```python
from build123d import *

# Parameters (mm, degrees)
SKETCH1_W           = 110.5916
SKETCH1_H           = 110.2233
BOSS_EXTRUDE1_DEPTH = 30.6832
SKETCH3_W           = 56.134
SKETCH3_H           = 21.0439
BOSS_EXTRUDE2_DEPTH = 2.54
SKETCH6_W           = 6.096
SKETCH6_H           = 6.1087
SKETCH6_W_2         = 6.1087
SKETCH6_H_2         = 6.096
SKETCH6_W_3         = 6.09854
SKETCH6_H_3         = 5.5245
BOSS_EXTRUDE3_DEPTH = 10.922


with BuildPart() as part:
    # Sketch1 → Boss-Extrude1 (new body)
    with BuildSketch(Plane.XY):
        Rectangle(SKETCH1_W, SKETCH1_H)
    extrude(amount=BOSS_EXTRUDE1_DEPTH)

    # Sketch3 → Boss-Extrude2 (add)
    with BuildSketch(Plane.XY.offset(30.6832)):
        with Locations((1.7018, 39.5097)):
            Rectangle(SKETCH3_W, SKETCH3_H)
    extrude(amount=BOSS_EXTRUDE2_DEPTH)

    # Sketch6 → Boss-Extrude3 (add)
    with BuildSketch(Plane.XY.offset(30.6832)):
        with Locations((-2.1971, 19.9517)):
            Rectangle(SKETCH6_W, SKETCH6_H)
        with Locations((-11.09345, 14.43355)):
            Rectangle(SKETCH6_W_2, SKETCH6_H_2)
        with Locations((6.71957, 14.43355)):
            Rectangle(SKETCH6_W_3, SKETCH6_H_2)
        with Locations((-2.1971, 11.81735)):
            Rectangle(SKETCH6_W, SKETCH6_H_2)
        with Locations((21.19884, 20.2438)):
            Rectangle(SKETCH6_W, SKETCH6_H_3)
        with Locations((21.2471, 11.81735)):
            Rectangle(SKETCH6_W, SKETCH6_H_2)
    extrude(amount=BOSS_EXTRUDE3_DEPTH)


solid = part.part
```
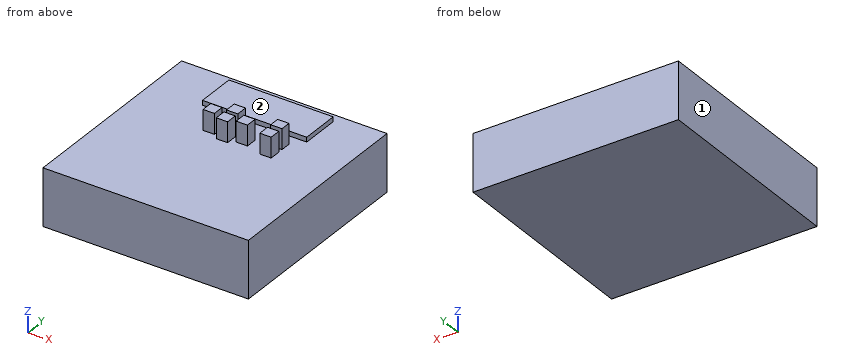
Model file for the job. Use its own axes, mm. Face numbers are marked on the shaded views. A direction names the side the tool comes from. Give positions to 0.01 mm unless a question says otherwise; leave off trailing zeros. Order: outer loops, then holes, each group sorted by start corner. A loop starts at its lowest first (then second) coordinate and runs counter-clockwise, first axis right, second up.
1) Saw through at A-A, the plane z = 37.5. Write the cut outline in (x, y).
2) Wall check: probe 1 along Z at (x, y) = (-45, 51); probe 2 along Z at (x, y) = (8, 36.5). Give the ranges that are in metal, low to high.
3) Saw through at C-C, the plane y = 40.5. Write the cut outline in (x, z).
4) 3-axis set-ups, long thin cutter, end or side, ignore diameter. For the marked faces 1 and 2: which of +Z, -Z, +X, -X, +Y, -Y reach the whole face in a straight line?
5) Saw through at B-B, the plane x = 8. Write the cut outline in (y, z), then the cut area to 3 significant figures.
6) Saw through at D-D, the plane x = -24.5. Write the cut outline in (y, z), then the cut area to 3 significant figures.
7) Pin check, flat tips, straight feed: pin 1 (17 mm diameter, centred on x = 15.5, y = 36, fed in from +Z); pin 2 (1.8 mm diameter, centred on x = -3, z = 36.5, fed in from -Y); pin 3 (3 mm diameter, centred on x = 21, z = 38.5, fed in from +Y). Stop position of each tip, or through.
Computed:
1. outline: (-14.15, 11.39) - (-8.04, 11.39) - (-8.04, 17.48) - (-14.15, 17.48) - close; (-5.25, 8.77) - (0.85, 8.77) - (0.85, 14.87) - (-5.25, 14.87) - close; (-5.25, 16.9) - (0.85, 16.9) - (0.85, 23.01) - (-5.25, 23.01) - close; (3.67, 11.39) - (9.77, 11.39) - (9.77, 17.48) - (3.67, 17.48) - close; (18.15, 17.48) - (24.25, 17.48) - (24.25, 23.01) - (18.15, 23.01) - close; (18.2, 8.77) - (24.3, 8.77) - (24.3, 14.87) - (18.2, 14.87) - close
2. probe 1: z = 0 to 30.68
2. probe 2: z = 0 to 33.22
3. outline: (-55.3, 0) - (55.3, 0) - (55.3, 30.68) - (29.77, 30.68) - (29.77, 33.22) - (-26.37, 33.22) - (-26.37, 30.68) - (-55.3, 30.68) - close
4. face 1: +Z, -Z, -X, +Y, -Y
4. face 2: +Z, +X, -X, +Y
5. outline: (-55.11, 0) - (55.11, 0) - (55.11, 30.68) - (50.03, 30.68) - (50.03, 33.22) - (28.99, 33.22) - (28.99, 30.68) - (17.48, 30.68) - (17.48, 41.61) - (11.39, 41.61) - (11.39, 30.68) - (-55.11, 30.68) - close
5. area: 3,500 mm2
6. outline: (-55.11, 0) - (55.11, 0) - (55.11, 30.68) - (50.03, 30.68) - (50.03, 33.22) - (28.99, 33.22) - (28.99, 30.68) - (-55.11, 30.68) - close
6. area: 3,440 mm2
7. pin 1: stops at z = 33.22
7. pin 2: stops at y = 8.77
7. pin 3: stops at y = 23.01
